The model under review builds one solid part; all positions refer to its coordinate system, in mm. Face numbers are marked on the shaded views. A direction names the side the tool comes from. Give positions to 0.01 mm unless a question says otherwise; leave off trailing zeros. Write each loop counter-clockwise with the first axis right and the second up, starting at its lowest first coordinate (ties: lowest second). Pieces come first, ordered by that corner, then holes. Notation, with made-up numbers: (35, 87.5) - (79, 87.5) arc R24 ccw to (79, 111.5) - close; hole circle Ø4 at (-37.5, 49). An arc over 180 degrees is marked (long way). Write item = value, one per line.
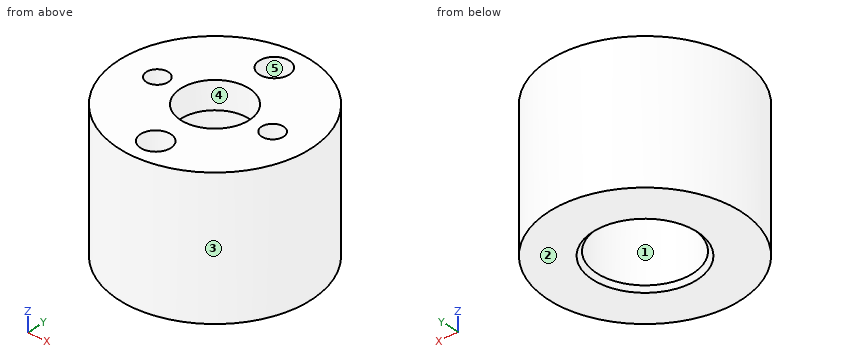
```python
from build123d import *

# Parameters (mm, degrees)
SKETCH2_R          = 2.5
CUT_EXTRUDE1_DEPTH = 13.727922061
SKETCH3_R          = 1.1
SKETCH3_R_2        = 0.8
CUT_EXTRUDE2_DEPTH = 2
CHAMFER1_SIZE      = 0.3


with BuildPart() as part:
    # Sketch1 → Revolve1 (revolve)
    with BuildSketch(Plane(origin=(0, 0, 0), x_dir=(1, 0, 0), z_dir=(0, 1, 0)), mode=Mode.PRIVATE) as revolve1_sk:
        Polygon((0, 0), (7, 0), (7, 10), (3.5, 10), (3.5, 2), (0, 2), align=None)
    revolve(revolve1_sk.sketch.rotate(Axis((0, 0, -2), (0, 0, 1)), 180), axis=Axis((0, 0, -2), (0, 0, 1)))

    # Sketch2 → Cut-Extrude1 (cut, through all)
    with BuildSketch(Plane(origin=(0, 0, -2), x_dir=(-1, 0, 0), z_dir=(0, 0, -1))):
        Circle(SKETCH2_R)
    extrude(amount=-CUT_EXTRUDE1_DEPTH, mode=Mode.SUBTRACT)

    # Sketch3 → Cut-Extrude2 (cut)
    with BuildSketch(Plane.XY):
        with Locations((0, 5)):
            Circle(SKETCH3_R)
        with Locations((0, -5)):
            Circle(SKETCH3_R)
        with Locations((4.25, 0)):
            Circle(SKETCH3_R_2)
        with Locations((-4.25, 0)):
            Circle(SKETCH3_R_2)
    extrude(amount=-CUT_EXTRUDE2_DEPTH, mode=Mode.SUBTRACT)

    # Chamfer1
    chamfer1_edges = [part.edges().sort_by_distance(p)[0] for p in [
        (3.5, 0, -10),
    ]]
    chamfer(chamfer1_edges, length=CHAMFER1_SIZE)


solid = part.part
```
1. Draft analysis for pull direction Y (two halves, no side actions). For the marked faces 1, 2 and 3, state which applies: +Y half, -Y half, draft (parallel to the pull), parting line (faces both ways), or undercut.
Findings below:
face_1 = undercut
face_2 = draft
face_3 = parting line
2. For line 1 (Y direction, x = -0.25, z = -7); line 2 (X direction, y = 1.25, z = -8.75), list the stretches that pass through material, from the lowest coordinate up. Write a range as from..to.
Findings below:
line_1 = -7..-3.49, 3.49..7
line_2 = -6.89..-3.27, 3.27..6.89
3. Insertion check: P1, Ø2, axis at x = 0, y = -5, coming from the +Z side; P2, Ø1.5, axis at y = -3.5, z = -8, coming from the +X side; P3, Ø1, axis at x = 3, z = -2, coming from the -Y side. Each pin has a flat end and moves straight along its axis. Give the tip position at first contact, or say it passes through.
Findings below:
P1 = -2
P2 = 6.44
P3 = -6.54
4. Take a section at B-B on y = 0. Give the boundary of the cut face in (x, z), and give its area (3 significant figures).
Findings below:
outline = (-7, -10) - (-3.8, -10) - (-3.5, -9.7) - (-3.5, -2) - (-5.05, -2) - (-5.05, 0) - (-7, 0) - close; (-3.45, -2) - (-2.5, -2) - (-2.5, 0) - (-3.45, 0) - close; (2.5, -2) - (3.45, -2) - (3.45, 0) - (2.5, 0) - close; (3.5, -9.7) - (3.8, -10) - (7, -10) - (7, 0) - (5.05, 0) - (5.05, -2) - (3.5, -2) - close
area = 67.5 mm²
5. Machinability: for the marked faces 4 and 5, which of the approach directions +Z, -Z, +X, -X, +Y, -Y give a long, thin tool a straight path to every point of the face, cutting with its end or side? Answer none if there is none.
Findings below:
face_4 = +Z, -Z
face_5 = +Z
6. Take a section at A-A on z = -1.75. Give the boundary of the cut face in (x, y), and give its area (3 significant figures).
Findings below:
outline = circle Ø14 at (0, 0); hole circle Ø1.6 at (-4.25, 0); hole circle Ø5 at (0, 0); hole circle Ø2.2 at (0, -5); hole circle Ø2.2 at (0, 5); hole circle Ø1.6 at (4.25, 0)
area = 123 mm²
7. Take a section at C-C on x = 0. Give the boundary of the cut face in (y, z), and give its area (3 significant figures).
Findings below:
outline = (-7, -10) - (-3.8, -10) - (-3.5, -9.7) - (-3.5, -2) - (-2.5, -2) - (-2.5, 0) - (-3.9, 0) - (-3.9, -2) - (-6.1, -2) - (-6.1, 0) - (-7, 0) - close; (2.5, -2) - (3.5, -2) - (3.5, -9.7) - (3.8, -10) - (7, -10) - (7, 0) - (6.1, 0) - (6.1, -2) - (3.9, -2) - (3.9, 0) - (2.5, 0) - close
area = 65.1 mm²
8. Take a section at D-D on x = 4.25. Give the boundary of the cut face in (y, z).
Findings below:
outline = (-5.56, -10) - (5.56, -10) - (5.56, 0) - (0.8, 0) - (0.8, -2) - (-0.8, -2) - (-0.8, 0) - (-5.56, 0) - close
